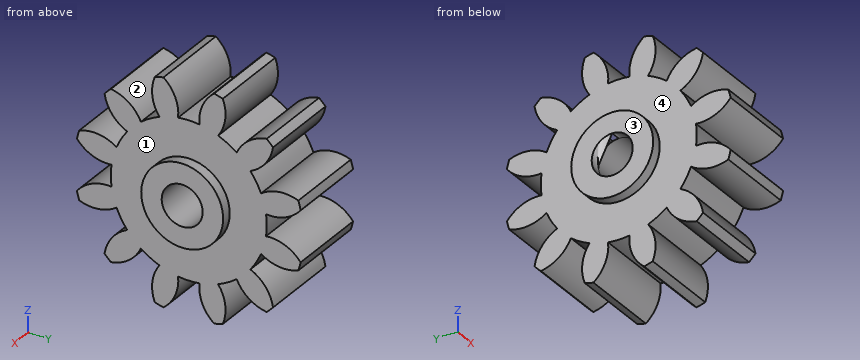
```python
from build123d import *

# Parameters (mm, degrees)
SPUR_START             = -44.990479754
SPUR_GEAR_AI_OUTLINE_R = 1.5875
SPUR_GEAR_AI_DEPTH     = 6.35
SKETCH1_R              = 3.175
SKETCH1_R_2            = 1.5875
BOSS_EXTRUDE1_DEPTH    = 0.8001
BOSS_EXTRUDE2_START    = 0.8001
SKETCH2_R              = 3.175
SKETCH2_R_2            = 1.5875
BOSS_EXTRUDE2_DEPTH    = 0.8001


# Read off the part's stored shape, not the designer's step: spur gear_ai
with BuildPart() as part:
    # spur gear_ai outline → spur gear_ai (new body)
    with BuildSketch(Plane.YZ.offset(SPUR_START)):
        with BuildLine():
            ThreePointArc((12.717986851, 12.671800633), (12.969814044, 12.913920885), (13.211934296, 13.165748078))
            ThreePointArc((13.211934296, 13.165748078), (12.629555475, 14.550963045), (11.456113125, 15.489588981))
            ThreePointArc((11.456113125, 15.489588981), (11.91893153, 16.17750017), (12.283270893, 16.92226826))
            ThreePointArc((12.283270893, 16.92226826), (13.682865973, 16.375350343), (15.173686734, 16.563602973))
            ThreePointArc((15.173686734, 16.563602973), (15.270715355, 16.899198858), (15.354484047, 17.238347731))
            ThreePointArc((15.354484047, 17.238347731), (14.15752171, 18.146789672), (12.671977858, 18.372942402))
            ThreePointArc((12.671977858, 18.372942402), (12.728834759, 19.20010017), (12.671977858, 20.027257937))
            ThreePointArc((12.671977858, 20.027257937), (14.15752171, 20.253410667), (15.354484047, 21.161852608))
            ThreePointArc((15.354484047, 21.161852608), (15.270715355, 21.501001481), (15.173686734, 21.836597366))
            ThreePointArc((15.173686734, 21.836597366), (13.682865973, 22.024849997), (12.283270893, 21.477932079))
            ThreePointArc((12.283270893, 21.477932079), (11.91893153, 22.222700169), (11.456113125, 22.910611358))
            ThreePointArc((11.456113125, 22.910611358), (12.629555475, 23.849237294), (13.211934296, 25.234452261))
            ThreePointArc((13.211934296, 25.234452261), (12.969814044, 25.486279454), (12.717986851, 25.728399706))
            ThreePointArc((12.717986851, 25.728399706), (11.332771884, 25.146020886), (10.394145948, 23.972578536))
            ThreePointArc((10.394145948, 23.972578536), (9.706234759, 24.43539694), (8.961466669, 24.799736303))
            ThreePointArc((8.961466669, 24.799736303), (9.508384586, 26.199331383), (9.320131956, 27.690152144))
            ThreePointArc((9.320131956, 27.690152144), (8.98453607, 27.787180765), (8.645387197, 27.870949457))
            ThreePointArc((8.645387197, 27.870949457), (7.736945256, 26.673987121), (7.510792527, 25.188443268))
            ThreePointArc((7.510792527, 25.188443268), (6.68363476, 25.24530017), (5.856476992, 25.188443268))
            ThreePointArc((5.856476992, 25.188443268), (5.630324262, 26.673987121), (4.721882321, 27.870949457))
            ThreePointArc((4.721882321, 27.870949457), (4.382733448, 27.787180765), (4.047137563, 27.690152144))
            ThreePointArc((4.047137563, 27.690152144), (3.858884932, 26.199331383), (4.405802849, 24.799736303))
            ThreePointArc((4.405802849, 24.799736303), (3.661034759, 24.43539694), (2.97312357, 23.972578536))
            ThreePointArc((2.97312357, 23.972578536), (2.034497635, 25.146020886), (0.649282668, 25.728399706))
            ThreePointArc((0.649282668, 25.728399706), (0.397455474, 25.486279454), (0.155335223, 25.234452261))
            ThreePointArc((0.155335223, 25.234452261), (0.737714043, 23.849237294), (1.911156393, 22.910611358))
            ThreePointArc((1.911156393, 22.910611358), (1.448337988, 22.222700169), (1.083998625, 21.477932079))
            ThreePointArc((1.083998625, 21.477932079), (-0.315596455, 22.024849997), (-1.806417216, 21.836597366))
            ThreePointArc((-1.806417216, 21.836597366), (-1.903445837, 21.501001481), (-1.987214529, 21.161852608))
            ThreePointArc((-1.987214529, 21.161852608), (-0.790252192, 20.253410667), (0.695291661, 20.027257937))
            ThreePointArc((0.695291661, 20.027257937), (0.638434759, 19.20010017), (0.695291661, 18.372942402))
            ThreePointArc((0.695291661, 18.372942402), (-0.790252192, 18.146789672), (-1.987214529, 17.238347731))
            ThreePointArc((-1.987214529, 17.238347731), (-1.903445837, 16.899198858), (-1.806417216, 16.563602973))
            ThreePointArc((-1.806417216, 16.563602973), (-0.315596455, 16.375350343), (1.083998625, 16.92226826))
            ThreePointArc((1.083998625, 16.92226826), (1.448337988, 16.17750017), (1.911156393, 15.489588981))
            ThreePointArc((1.911156393, 15.489588981), (0.737714043, 14.550963045), (0.155335223, 13.165748078))
            ThreePointArc((0.155335223, 13.165748078), (0.397455474, 12.913920884), (0.649282668, 12.671800633))
            ThreePointArc((0.649282668, 12.671800633), (2.034497635, 13.254179453), (2.97312357, 14.427621803))
            ThreePointArc((2.97312357, 14.427621803), (3.661034759, 13.964803399), (4.405802849, 13.600464036))
            ThreePointArc((4.405802849, 13.600464036), (3.858884932, 12.200868956), (4.047137563, 10.710048195))
            ThreePointArc((4.047137563, 10.710048195), (4.382733448, 10.613019574), (4.721882321, 10.529250882))
            ThreePointArc((4.721882321, 10.529250882), (5.630324262, 11.726213218), (5.856476992, 13.211757071))
            ThreePointArc((5.856476992, 13.211757071), (6.68363476, 13.15490017), (7.510792527, 13.211757071))
            ThreePointArc((7.510792527, 13.211757071), (7.736945256, 11.726213218), (8.645387197, 10.529250882))
            ThreePointArc((8.645387197, 10.529250882), (8.98453607, 10.613019574), (9.320131956, 10.710048195))
            ThreePointArc((9.320131956, 10.710048195), (9.508384586, 12.200868956), (8.961466669, 13.600464036))
            ThreePointArc((8.961466669, 13.600464036), (9.706234759, 13.964803399), (10.394145948, 14.427621803))
            ThreePointArc((10.394145948, 14.427621803), (11.332771884, 13.254179453), (12.717986851, 12.671800633))
        make_face()
        with Locations((6.683634759, 19.20010017)):
            Circle(SPUR_GEAR_AI_OUTLINE_R, mode=Mode.SUBTRACT)
    extrude(amount=SPUR_GEAR_AI_DEPTH)

    # Sketch1 → Boss-Extrude1 (add)
    with BuildSketch(Plane(origin=(-38.640479754, 0, 0), x_dir=(0, 0, -1), z_dir=(1, 0, 0))):
        with Locations(Location((-19.20010017, 6.683634759, 0), (0, 0, 180))):
            Circle(SKETCH1_R)
        with Locations((-19.20010017, 6.683634759)):
            Circle(SKETCH1_R_2, mode=Mode.SUBTRACT)
    extrude(amount=BOSS_EXTRUDE1_DEPTH)

    # Sketch2 → Boss-Extrude2 (add)
    with BuildSketch(Plane.ZY.offset(44.990479754).offset(BOSS_EXTRUDE2_START)):
        with Locations((19.20010017, 6.683634759)):
            Circle(SKETCH2_R)
        with Locations((19.20010017, 6.683634759)):
            Circle(SKETCH2_R_2, mode=Mode.SUBTRACT)
    extrude(amount=-BOSS_EXTRUDE2_DEPTH)


solid = part.part
```
Input: part model. Units: mm. Frame: model coordinates. Face numbers are marked on the shaded views. A direction names the side the tool comes from. Round coordinates to 2 decimals unless told otherwise and drop trailing zeros. Loops run counter-clockwise (first coordinate to the right, second up) from the corner with the lowest first, then second, coordinate; pieces in that order, holes last. Notation, with made-up numbers: (42.25, -27) - (52.25, -27) arc R23 cw to (52.25, -19) - close; hole circle Ø2 at (44.25, 9). An arc over 180 degrees is marked (long way). One line per item, written item: value. Start each with the question number.
(1) Ray query, line 1 (Y direction, x = -40, z = 24.5); line 2 (X direction, y = 10, z = 17.25); line 3 (Y direction, x = -44.5, z = 17.75). Return the intervals inside material, ascending. Write a range as [from, to].
(2) Access query for the marked faces 3 and 4. Directions: +Z, -Z, +X, -X, +Y, -Y. A direction counts if a zero-diameter tool reaches every point of the face in a straight line with its end or side. Return the directions, or none.
(3) Draft query along Y for the marked faces 1 and 2. Return one class per face: +Y half, -Y half, draft (parallel to the pull), parting line (faces both ways), or undercut.
(4) Contact query for flat-ended pins moving along their axis: P1, Ø2, axis at x = -42, y = 13.5, coming from the -Z side; P2, Ø1, axis at x = -39, z = 15, coming from the -Y side; P3, Ø2, axis at x = -45, z = 24, coming from the +Y side. Output: stop coordinate, or through.
(5) Section D-D, the plane y = 13. Return loops of the section in (x, z).
(6) Section B-B, the plane y = 5.5. Return loops of the section in (x, z).
(7) Section A-A, the plane z = 25.5. Return loops of the section in (x, y).
Results below:
1. line 1: [0.36, 2.67], [3.78, 9.59], [10.7, 13.01]
1. line 2: [-44.99, -38.64]
1. line 3: [-1.47, 6.04], [7.33, 14.84]
2. face 3: +Z, -Z, -X, +Y, -Y
2. face 4: -X
3. face 1: draft
3. face 2: undercut
4. P1: z = 12.67
4. P2: y = 0.7
4. P3: y = 13.17
5. outline: (-44.99, 12.94) - (-38.64, 12.94) - (-38.64, 13.91) - (-44.99, 13.91) - close; (-44.99, 16.54) - (-38.64, 16.54) - (-38.64, 18.39) - (-44.99, 18.39) - close; (-44.99, 20.01) - (-38.64, 20.01) - (-38.64, 21.86) - (-44.99, 21.86) - close; (-44.99, 24.49) - (-38.64, 24.49) - (-38.64, 25.46) - (-44.99, 25.46) - close
6. outline: (-45.79, 16.25) - (-44.99, 16.25) - (-44.99, 11.46) - (-38.64, 11.46) - (-38.64, 16.25) - (-37.84, 16.25) - (-37.84, 18.14) - (-45.79, 18.14) - close; (-45.79, 20.26) - (-37.84, 20.26) - (-37.84, 22.15) - (-38.64, 22.15) - (-38.64, 26.94) - (-44.99, 26.94) - (-44.99, 22.15) - (-45.79, 22.15) - close
7. outline: (-44.99, 0.41) - (-38.64, 0.41) - (-38.64, 1.43) - (-44.99, 1.43) - close; (-44.99, 4.03) - (-38.64, 4.03) - (-38.64, 5.87) - (-44.99, 5.87) - close; (-44.99, 7.5) - (-38.64, 7.5) - (-38.64, 9.34) - (-44.99, 9.34) - close; (-44.99, 11.93) - (-38.64, 11.93) - (-38.64, 12.96) - (-44.99, 12.96) - close
